Model file for the job. Use its own axes, mm. A direction names the side the tool comes from. Give positions to 0.01 mm unless a question says otherwise; leave off trailing zeros. Write each loop counter-clockwise with the first axis right and the second up, starting at its lowest first coordinate (ties: lowest second). Pieces come first, ordered by that corner, then holes. Notation, with made-up numbers: (56.25, 83) - (94.25, 83) arc R18 cw to (94.25, 97) - close; hole circle Ø7 at (57, -13). An arc over 180 degrees is marked (long way). Use a Markdown table: item, result. Add a question column.
```python
from build123d import *

# Parameters (mm, degrees)
F0_W     = 38.225519
F0_H     = 68.893833
F1_DEPTH = 5
F2_W     = 100
F2_H     = 24.910029
F3_DEPTH = 5
F4_R     = 1.85
F5_DEPTH = 25.4
F6_W     = 25
F6_H     = 20
F7_DEPTH = 10
F8_R     = 3.25
F9_DEPTH = 5


with BuildPart() as f1:
    # F0 (on Top) → F1 (new body)
    with BuildSketch(Plane.XY):
        with Locations((4.975074, 16.320151)):
            Rectangle(F0_W, F0_H)
    extrude(amount=-F1_DEPTH)

    # F2 (on face) → F3 (join)
    with BuildSketch(Plane(origin=(0, 0, -5), x_dir=(1, 0, 0), z_dir=(0, 0, -1))):
        with Locations((5.092296, -18.559826)):
            Rectangle(F2_W, F2_H)
    extrude(amount=-F3_DEPTH)

    # F4 (on face) → F5 (cut)
    with BuildSketch(Plane.XY):
        with Locations((-41.387634, 27.575926)):
            Circle(F4_R)
        with Locations((51.599746, 27.514396)):
            Circle(F4_R)
        with Locations((-41.413683, 9.564399)):
            Circle(F4_R)
        with Locations((51.624972, 9.70294)):
            Circle(F4_R)
    extrude(amount=-F5_DEPTH, mode=Mode.SUBTRACT)

    # F6 (on face) → F7 (join)
    with BuildSketch(Plane(origin=(0, 0, -5), x_dir=(1, 0, 0), z_dir=(0, 0, -1))):
        with Locations((4.862315, 4.593138)):
            Rectangle(F6_W, F6_H)
    extrude(amount=F7_DEPTH)

    # F8 (on face) → F9 (cut)
    with BuildSketch(Plane(origin=(0, 0, -15), x_dir=(1, 0, 0), z_dir=(0, 0, -1))):
        with Locations((4.862315, 4.593138)):
            Circle(F8_R)
    extrude(amount=-F9_DEPTH, mode=Mode.SUBTRACT)


solid = f1.part
```
(1) Band-saw the part on D-D (z = -8). Write the cut outline in (x, y).
(2) Flat gauge pins, fed straight in: pin 1 (4 mm diameter, centred on x = -28, z = -3, fed in from +Y); pin 2 (4 mm diameter, centred on y = 46, z = -2.5, fed in from +X); pin 3 (3 mm diameter, centred on x = 51.62, y = 9.7, fed in from -Z); pin 4 (20.5 mm diameter, centred on x = 17, y = 17, fed in from -Z). Where does each tip first touch, or does it go through?
(3) Which spindle directions (+Z, -Z, +X, -X, +Y, -Y) get a long thin tool onto all of the face, cutting with end or side? Do faces 1 (the flat face through (24.088, -6, -2)), 2 (the flat face through (-30, 31.015, -3)), 3 (the flat face through (-14.138, -6, -2)). Say none if no direction does.
(4) Band-saw the part on A-A (y = 4). Write the cut outline in (x, z), then the cut area to 3 significant figures.
(5) Two-plate mould, pull along X, no slides. Class faces 4 (the cylindrical face through (-39.65, 10.12, -2.46)), 5 (the flat face through (55.092, 19, -3)), 6 (the flat face through (5, -18.127, -2)): +X half, -X half, draft (parallel to the pull), parting line (faces both ways), or undercut.
(6) Band-saw the part on B-B (z = -3.5). Write the cut outline in (x, y), then the cut area to 3 significant figures.
(7) Probe probe 1 along X at (y, z) = (27.5, -3); probe 2 along Z at (x, y) = (-38.5, 12.5); probe 3 along Y at (x, z) = (46, -3.5). List the from-to ranges inside material, lowest first. Write a range as [from, to].
(8) Band-saw the part on C-C (x = 11). Write the cut outline in (y, z).
Model answer:
| question | item | result |
|---|---|---|
| 1 | outline | (-7.64, -14.59) - (17.36, -14.59) - (17.36, 5.41) - (-7.64, 5.41) - close |
| 2 | pin 1 | stops at y = 31.01 |
| 2 | pin 2 | stops at x = 24.09 |
| 2 | pin 3 | passes through |
| 2 | pin 4 | stops at z = -5 |
| 3 | face 1 | +Z, -Z, +X, -Y |
| 3 | face 2 | +Z, -Z, -X, +Y |
| 3 | face 3 | +Z, -Z, -X, -Y |
| 4 | outline | (-14.14, -5) - (-7.64, -5) - (-7.64, -15) - (17.36, -15) - (17.36, -5) - (24.09, -5) - (24.09, 0) - (-14.14, 0) - close |
| 4 | area | 441 mm^2 |
| 5 | face 4 | undercut |
| 5 | face 5 | +X half |
| 5 | face 6 | draft |
| 6 | outline | (-44.91, 6.1) - (-14.14, 6.1) - (-14.14, -18.13) - (24.09, -18.13) - (24.09, 6.1) - (55.09, 6.1) - (55.09, 31.01) - (24.09, 31.01) - (24.09, 50.77) - (-14.14, 50.77) - (-14.14, 31.01) - (-44.91, 31.01) - close; hole circle Ø3.7 at (-41.41, 9.56); hole circle Ø3.7 at (-41.39, 27.58); hole circle Ø3.7 at (51.6, 27.51); hole circle Ø3.7 at (51.62, 9.7) |
| 6 | area | 4,130 mm^2 |
| 7 | probe 1 | x = [-44.91, -43.24], [-39.54, 49.75], [53.45, 55.09] |
| 7 | probe 2 | z = [-5, 0] |
| 7 | probe 3 | y = [6.1, 31.01] |
| 8 | outline | (-18.13, -5) - (-14.59, -5) - (-14.59, -15) - (5.41, -15) - (5.41, -5) - (50.77, -5) - (50.77, 0) - (-18.13, 0) - close |
